Design review of the part built by this model. Coordinates are the model's own, in mm. Face numbers are marked on the shaded views. A direction names the side the tool comes from. Coordinates: 2 decimals unless noted, no trailing zeros. Write each loop counter-clockwise with the first axis right and the second up, starting at its lowest first coordinate (ties: lowest second). Pieces come first, ordered by that corner, then holes.
Q1. Take a section at C-C, the plane y = 5.5. Write out the cut boundary in (x, z).
Q2. For the marked faces 1 and 2, list the 3-axis set-ups (+Z, -Z, +X, -X, +Y, -Y) from which the entire face can be reached by the end or side of a thin tool; tool diameter is ignored.
Q3. Take a section at B-B, the plane x = -5.75. Write out the cut boundary in (y, z).
Q4. For L1, parallel to X at y = 14.75, z = 1.25; L2, parallel to X at y = 17.5, z = 2; L3, parallel to Y at x = -6.5, z = 4.25, list the stretches that pass through material, from the lowest coordinate up.
Q5. Take a section at A-A, the plane z = 5.5. Write out the cut boundary in (x, y), plus the area to 3 significant figures.
Q6. For pin 1 Ø3 at (x, z) = (-5.5, 5.5) entering from -Y; pin 2 Ø1.2 at (x, z) = (-6, 3.5) entering from -Y, all flat-tipped, find the tip position at first contact; note any pin that passes through.
Q7. The part is to be moulded in two halves that separate along X. For the marked faces 3, 4 and 5, say which applies: released by +X, released by -X, zero draft, split by the parting line, or undercut.
from build123d import *

# Parameters (mm, degrees)
F1_DEPTH = 10
F2_R     = 3


with BuildPart() as f1:
    # F0 (on Top) → F1 (new body)
    with BuildSketch(Plane.XY):
        with BuildLine():
            ThreePointArc((-9.581522, 0), (-8.167308, 0.585786), (-7.581522, 2))
            Line((-7.581522, 2), (-7.581522, 19.23404))
            Line((-7.581522, 19.23404), (-5.081522, 19.23404))
            Line((-5.081522, 19.23404), (-3.581522, 16.635963))
            ThreePointArc((-3.581522, 16.635963), (-2.367109, 15.704112), (-0.849471, 15.903913))
            Line((-0.849471, 15.903913), (-0.416458, 16.153913))
            Line((-0.416458, 16.153913), (-3.638146, 21.73404))
            Line((-3.638146, 21.73404), (-10.081522, 21.73404))
            Line((-10.081522, 21.73404), (-10.081522, 0))
            Line((-10.081522, 0), (-9.581522, 0))
        make_face()
    extrude(amount=F1_DEPTH)

    # F2
    f2_edges = [f1.edges().sort_by_distance(p)[0] for p in [
        (-3.638146, 21.73404, 5),
    ]]
    fillet(f2_edges, radius=F2_R)


solid = f1.part
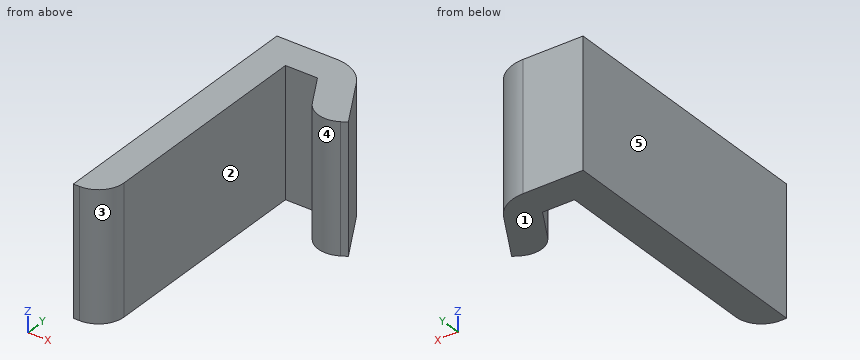
Responses:
1. outline: (-10.08, 0) - (-7.58, 0) - (-7.58, 10) - (-10.08, 10) - close
2. face 1: -Z, +X, -X, +Y, -Y
2. face 2: +Z, -Z, -Y
3. outline: (19.23, 0) - (21.73, 0) - (21.73, 10) - (19.23, 10) - close
4. L1: x = -10.08 to -7.58
4. L2: x = -10.08 to -7.58, -4.08 to -1.19
4. L3: y = 19.23 to 21.73
5. outline: (-10.08, 0) - (-9.58, 0) arc R2 ccw to (-7.58, 2) - (-7.58, 19.23) - (-5.08, 19.23) - (-3.58, 16.64) arc R2 ccw to (-0.85, 15.9) - (-0.42, 16.15) - (-2.77, 20.23) arc R3 ccw to (-5.37, 21.73) - (-10.08, 21.73) - close
5. area: 74.5 mm2
6. pin 1: stops at y = 17.36
6. pin 2: stops at y = 19.23
7. face 3: released by +X
7. face 4: undercut
7. face 5: released by -X
